from build123d import *

# Parameters (mm, degrees)
BOSS_EXTRUDE1_DEPTH = 34.2
SKETCH2_R           = 1.75
SKETCH2_R_2         = 3
CUT_EXTRUDE2_DEPTH  = 4
SKETCH3_R           = 10.5
CUT_EXTRUDE3_DEPTH  = 1
SKETCH5_R           = 1.75
CUT_EXTRUDE7_DEPTH  = 4
FILLET2_R           = 3
FILLET3_R           = 3
SKETCH12_R          = 2.595
CUT_EXTRUDE8_DEPTH  = 4
SKETCH14_W          = 17.1
SKETCH14_H          = 6
CUT_EXTRUDE9_DEPTH  = 4
SKETCH15_R          = 3
BOSS_EXTRUDE2_DEPTH = 10


with BuildPart() as part:
    # Sketch1 → Boss-Extrude1 (new body)
    with BuildSketch(Plane(origin=(0, 0, 0), x_dir=(1, 0, 0), z_dir=(0, 1, 0))):
        Polygon((0, 0), (34.2, 0), (41.271067812, -7.071067812), (51.271067812, -7.071067812), (51.271067812, -26.928932188), (41.271067812, -26.928932188), (34.2, -34), (0, -34), (0, -38), (34.2, -38), (41.271067812, -30.928932188), (55.271067812, -30.928932188), (55.271067812, -26.928932188), (55.271067812, -3.071067812), (51.271067812, -3.071067812), (41.271067812, -3.071067812), (34.2, 4), (0, 4), align=None)
    extrude(amount=BOSS_EXTRUDE1_DEPTH)

    # Sketch2 → Cut-Extrude2 (cut)
    with BuildSketch(Plane(origin=(0, 0, -4), x_dir=(-1, 0, 0), z_dir=(0, 0, -1))):
        with Locations((-28.675, 28.675)):
            Circle(SKETCH2_R)
        with Locations((-5.525, 28.675)):
            Circle(SKETCH2_R)
        with Locations((-5.525, 5.525)):
            Circle(SKETCH2_R)
        with Locations((-28.675, 5.525)):
            Circle(SKETCH2_R)
        with Locations((-17.1, 17.1)):
            Circle(SKETCH2_R_2)
    extrude(amount=-CUT_EXTRUDE2_DEPTH, mode=Mode.SUBTRACT)

    # Sketch3 → Cut-Extrude3 (cut)
    with BuildSketch(Plane.XY):
        with Locations((17.1, 17.1)):
            Circle(SKETCH3_R)
    extrude(amount=-CUT_EXTRUDE3_DEPTH, mode=Mode.SUBTRACT)

    # Sketch5 → Cut-Extrude7 (cut)
    with BuildSketch(Plane.XY.offset(38)):
        with Locations((28.675, 28.675)):
            Circle(SKETCH5_R)
        with Locations((5.525, 28.675)):
            Circle(SKETCH5_R)
        with Locations((5.525, 5.525)):
            Circle(SKETCH5_R)
        with Locations((28.675, 5.525)):
            Circle(SKETCH5_R)
    extrude(amount=-CUT_EXTRUDE7_DEPTH, mode=Mode.SUBTRACT)

    # Fillet2
    fillet2_edges = [part.edges().sort_by_distance(p)[0] for p in [
        (0, 0, 36),
        (0, 0, -2),
        (0, 34.2, 36),
        (0, 34.2, -2),
    ]]
    fillet(fillet2_edges, radius=FILLET2_R)

    # Fillet3
    fillet3_edges = [part.edges().sort_by_distance(p)[0] for p in [
        (55.271067812, 17.1, 3.071067812),
        (55.271067812, 17.1, 30.928932188),
    ]]
    fillet(fillet3_edges, radius=FILLET3_R)

    # Sketch12 → Cut-Extrude8 (cut)
    with BuildSketch(Plane(origin=(55.271067812, 0, 0), x_dir=(0, 0, -1), z_dir=(1, 0, 0))):
        with Locations((-17, 17.1)):
            Circle(SKETCH12_R)
    extrude(amount=-CUT_EXTRUDE8_DEPTH, mode=Mode.SUBTRACT)

    # Sketch14 → Cut-Extrude9 (cut)
    with BuildSketch(Plane(origin=(0, 0, -4), x_dir=(-1, 0, 0), z_dir=(0, 0, -1))):
        with Locations((-8.55, 17.1)):
            Rectangle(SKETCH14_W, SKETCH14_H)
    extrude(amount=-CUT_EXTRUDE9_DEPTH, mode=Mode.SUBTRACT)

    # Sketch15 → Boss-Extrude2 (add)
    with BuildSketch(Plane.XY.offset(38)):
        with Locations((17.086482483, 17.08469774)):
            Circle(SKETCH15_R)
    extrude(amount=BOSS_EXTRUDE2_DEPTH)


solid = part.part
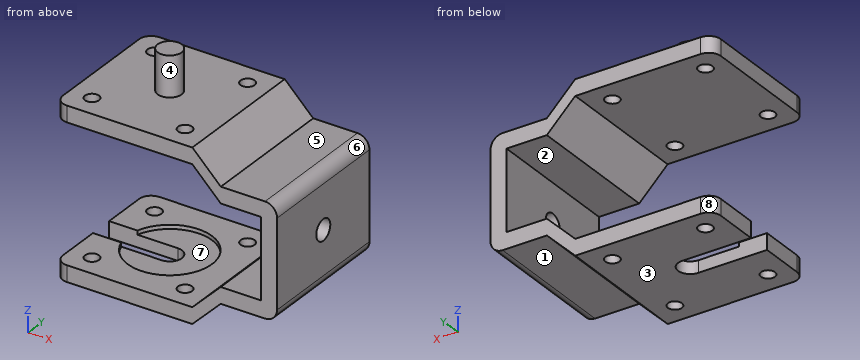
Here's how the part is built. I have some questions about the finished solid (model axes, mm). Face numbers are marked on the shaded views. A direction names the side the tool comes from. Coordinates: 2 decimals unless noted, no trailing zeros. Write each loop counter-clockwise with the first axis right and the second up, starting at its lowest first coordinate (ties: lowest second). Pieces come first, ordered by that corner, then holes.
Item 1: I want a section at A-A on z = 17. Write out the boundary of the cut face in (x, y) (3 decimals).
Item 2: If we mould it in two halves opening along Y, with no side actions, what happens to the marked faces 6, 7 and 8? For each: +Y half, -Y half, draft (parallel to the pull), parting line (faces both ways), or undercut.
Item 3: I want a section at D-D on z = 44.5. Write out the boundary of the cut face in (x, y), and give its area (3 significant figures).
Item 4: I want a section at C-C on z = 32. Write out the boundary of the cut face in (x, y).
Item 5: On a 3-axis mill with a long thin cutter (end or side, diameter ignored), from which of +Z, -Z, +X, -X, +Y, -Y can I reach the whole of each face in a straight line? I mean the marked faces 1, 2, 3, 4 and 5. Say none if no direction works.
Item 6: Will these pins go through, and if not, where does the flat tip stop? pin 1 (5.5 mm diameter, centred on x = 46.5, y = 11.5, fed in from -Z); pin 2 (3 mm diameter, centred on x = 34.5, y = 4, fed in from +Z); pin 3 (10.5 mm diameter, centred on x = 24.5, y = 19, fed in from +Z); pin 4 (6 mm diameter, centred on y = 13, z = 17.5, fed in from -X).
Item 7: I want a section at B-B on x = 33.5. Write out the boundary of the cut face in (y, z).
Item 8: If I drill on line 1 (Z direction, x = 17.5, y = 27); line 2 (Z direction, x = 43.5, y = 27); line 3 (X direction, y = 30, z = 37.5), over which ranges is the centre line in solid material (lowest first)?
Findings below:
1. outline: (51.271, 0) - (55.271, 0) - (55.271, 14.505) - (51.271, 14.505) - close; (51.271, 19.695) - (55.271, 19.695) - (55.271, 34.2) - (51.271, 34.2) - close
2. face 6: draft
2. face 7: undercut
2. face 8: +Y half
3. outline: circle Ø6 at (17.09, 17.08)
3. area: 28.3 mm2
4. outline: (36.2, 0) - (40.2, 0) - (40.2, 34.2) - (36.2, 34.2) - close
5. face 1: -Z, +X, +Y, -Y
5. face 2: -X, +Y, -Y
5. face 3: -Z, +X, -X, +Y, -Y
5. face 4: +Z
5. face 5: +Z, +X, +Y, -Y
6. pin 1: stops at z = 3.07
6. pin 2: stops at z = 38
6. pin 3: stops at z = 48
6. pin 4: stops at x = 51.27
7. outline: (0, -4) - (34.2, -4) - (34.2, 0) - (0, 0) - close; (0, 34) - (34.2, 34) - (34.2, 38) - (0, 38) - close
8. line 1: z = -4 to -1, 34 to 38
8. line 2: z = 3.07 to 7.07, 26.93 to 30.93
8. line 3: x = 0 to 4.38, 6.67 to 27.53, 29.82 to 34.7
